Geometry: final body of the model. Coordinates: model frame, mm. A direction names the side the tool comes from. Give positions to 0.01 mm unless a question says otherwise; leave off trailing zeros. Write each loop counter-clockwise with the first axis right and the second up, starting at its lowest first coordinate (ties: lowest second). Pieces come first, ordered by that corner, then holes.
```python
from build123d import *

# Parameters (mm, degrees)
SKETCH1_W           = 12.192
SKETCH1_H           = 24.384
BOSS_EXTRUDE1_DEPTH = 5.4356
SKETCH2_W           = 3.7465
SKETCH2_H           = 5.4356
CUT_EXTRUDE1_DEPTH  = 5.4356
SKETCH3_W           = 1.905
SKETCH3_H           = 2.794
BOSS_EXTRUDE2_DEPTH = 5.4356
SKETCH4_W           = 1.27
SKETCH4_H           = 21.7424
BOSS_EXTRUDE3_DEPTH = 5.4356
SKETCH5_W           = 3.175
SKETCH5_H           = 0.254
SKETCH5_W_2         = 1.905
SKETCH5_W_3         = 8.382
CUT_EXTRUDE2_DEPTH  = 31.279271711


with BuildPart() as part:
    # Sketch1 → Boss-Extrude1 (new body)
    with BuildSketch(Plane.XY):
        with Locations((6.096, 12.192)):
            Rectangle(SKETCH1_W, SKETCH1_H)
    extrude(amount=BOSS_EXTRUDE1_DEPTH)

    # Sketch2 → Cut-Extrude1 (cut)
    with BuildSketch(Plane.XY.offset(5.4356)):
        with Locations((1.87325, 2.7178)):
            Rectangle(SKETCH2_W, SKETCH2_H)
        with Locations((10.31875, 2.7178)):
            Rectangle(SKETCH2_W, SKETCH2_H)
    extrude(amount=-CUT_EXTRUDE1_DEPTH, mode=Mode.SUBTRACT)

    # Sketch3 → Boss-Extrude2 (add)
    with BuildSketch(Plane.XY.offset(5.4356)):
        with Locations((0.9525, 25.781)):
            Rectangle(SKETCH3_W, SKETCH3_H)
        with Locations((11.2395, 25.781)):
            Rectangle(SKETCH3_W, SKETCH3_H)
    extrude(amount=-BOSS_EXTRUDE2_DEPTH)

    # Sketch4 → Boss-Extrude3 (add)
    with BuildSketch(Plane.XY.offset(5.4356)):
        with Locations((-0.635, 16.3068)):
            Rectangle(SKETCH4_W, SKETCH4_H)
    extrude(amount=-BOSS_EXTRUDE3_DEPTH)

    # Sketch5 → Cut-Extrude2 (cut, through all)
    with BuildSketch(Plane.XY.offset(5.4356)):
        with Locations((0.3175, 27.051)):
            Rectangle(SKETCH5_W, SKETCH5_H)
        with Locations((11.2395, 27.051)):
            Rectangle(SKETCH5_W_2, SKETCH5_H)
        with Locations((6.096, 24.257)):
            Rectangle(SKETCH5_W_3, SKETCH5_H)
    extrude(amount=-CUT_EXTRUDE2_DEPTH, mode=Mode.SUBTRACT)


solid = part.part
```
Item 1: Section A-A, the plane z = 0.9. Return the cut outline in (x, y) (1 decimal), plus the area to 3 significant figures.
Found:
outline: (-1.3, 5.4) - (3.7, 5.4) - (3.7, 0) - (8.4, 0) - (8.4, 5.4) - (12.2, 5.4) - (12.2, 26.9) - (10.3, 26.9) - (10.3, 24.1) - (1.9, 24.1) - (1.9, 26.9) - (-1.3, 26.9) - close
area: 291 mm2
Item 2: Reachability of faces 4 (the face through (3.746, 3, 3)), 5 (the face through (-1.27, 16, 3)), 6 (the face through (6, 24.13, 3)), 7 (the face through (10, 5.436, 3)), 8 (the face through (11, 26.924, 3)) from +Z, -Z, +X, -X, +Y, -Y: full face, straight path, thin tool, end or side. Return the list, or none.
Found:
face 4: +Z, -Z, -X, -Y
face 5: +Z, -Z, -X, +Y, -Y
face 6: +Z, -Z, +Y
face 7: +Z, -Z, +X, -Y
face 8: +Z, -Z, +X, -X, +Y
Item 3: Line query: L1, parallel to X at y = 25.25, z = 4.8 (3 decimals); L2, parallel to Y at x = 3.25, z = 1.8; L3, parallel to Y at x = 1, z = 2.75. Output: solid intervals per line, ascending.
Found:
L1: x = -1.27 to 1.905, 10.287 to 12.192
L2: y = 5.44 to 24.13
L3: y = 5.44 to 26.92
Item 4: Section C-C, the plane x = 11. Return the cut outline in (y, z), plus the area to 3 significant figures.
Found:
outline: (5.44, 0) - (26.92, 0) - (26.92, 5.44) - (5.44, 5.44) - close
area: 117 mm2
Item 5: Pull-direction query (X, two-part tool) for faces 1 (the face through (8.446, 3, 3)), 2 (the face through (10.287, 26, 3)), 3 (the face through (5, 14, 5.436)); classes: +X half, -X half, draft (parallel to the pull), parting line (faces both ways), or undercut.
Found:
face 1: +X half
face 2: undercut
face 3: draft
Item 6: Section B-B, the plane x = 5. Return the cut outline in (y, z), plus the area to 3 significant figures.
Found:
outline: (0, 0) - (24.13, 0) - (24.13, 5.44) - (0, 5.44) - close
area: 131 mm2
Item 7: Pin query (flat end, axial travel): pin 1 Ø1.5 at (x, z) = (10, 3.5) entering from -Y; pin 2 Ø2.5 at (x, z) = (4, 3) entering from +Y. Return the tip coordinate at first contact, or that it passes through.
Found:
pin 1: stops at y = 5.44
pin 2: stops at y = 24.13
